Could you check a few things on this model? Use its own coordinates, in mm. A direction names the side the tool comes from. Give positions to 0.01 mm unless a question says otherwise; leave off trailing zeros. Write each loop counter-clockwise with the first axis right and the second up, starting at its lowest first coordinate (ties: lowest second). Pieces come first, ordered by that corner, then holes. Notation, with made-up numbers: M 24.25,-5 L 75.25,-5 A23 ccw 75.25,3 Z; hole C 88.5,-5 d3. An arc over 180 degrees is marked long. Answer as a JSON object with one key per item and string values. Group by question number.
```python
from build123d import *

# Parameters (mm, degrees)
F0_R        = 10.16
F1_DEPTH    = 3.81
F2_R        = 12.7
F3_DEPTH    = 2.54
F4_R        = 11.43
F5_DEPTH    = 38.1
F6_S5_R     = 12.7
F6_T6_DEPTH = 25
F7_W        = 12.7
F7_H        = 12.7
F8_DEPTH    = 16.51
F9_W        = 12.7
F9_H        = 12.7
F10_DEPTH   = 16.51


# Not quite as in the source:
# - a fillet or chamfer that OpenCascade refuses, or shapes differently, is made with other operations: its cross-section is extruded or revolved along the edge and cut away or added


with BuildPart() as f1:
    # F0 (on Top) → F1 (new body)
    with BuildSketch(Plane.XY):
        Circle(F0_R)
    extrude(amount=-F1_DEPTH)

    # F2 (on Top) → F3 (join)
    with BuildSketch(Plane.XY):
        Circle(F2_R)
    extrude(amount=F3_DEPTH)

    # F4 (on Top) → F5 (join)
    with BuildSketch(Plane.XY):
        Circle(F4_R)
    extrude(amount=F5_DEPTH)

    # F6: chamfer of 5.08 on 3 edges, made by hand


with BuildPart() as f6_tool2:
    # F6_s3 → F6_t4 (revolve)
    with BuildSketch(Plane.XZ):
        Polygon((16.51, 2.54), (11.43, 7.62), (11.43, 2.54), align=None)
    revolve(axis=Axis((0, 0, 2.54), (0, 0, -1)))

    # F6_s5 → F6_t6 (intersect, symmetric)
    with BuildSketch(Plane.XY.offset(5.1)):
        Circle(F6_S5_R)
    extrude(amount=F6_T6_DEPTH, both=True, mode=Mode.INTERSECT)


with BuildPart() as f1_1:
    add(f1.part)

    # F6_t1: union F6_tool2
    add(f6_tool2.part)

    # F6_s7 → F6_t8 (revolve, cut)
    with BuildSketch(Plane.XZ):
        Polygon((11.43, 33.02), (6.35, 38.1), (11.43, 38.1), align=None)
    revolve(axis=Axis((0, 0, 38.1), (0, 0, 1)), mode=Mode.SUBTRACT)

    # F7 (on Right) → F8 (join)
    with BuildSketch(Plane.YZ):
        with Locations((0, 19.9612583965)):
            Rectangle(F7_W, F7_H)
    extrude(amount=F8_DEPTH)

    # F9 (on Right) → F10 (join)
    with BuildSketch(Plane.YZ):
        with Locations((0, 19.9612583965)):
            Rectangle(F9_W, F9_H)
    extrude(amount=-F10_DEPTH)


solid = f1_1.part
```
1) If we section it at C-C, the plane z = 5.5: List the corners of the cut face in (x, y) for me, plus the area to 3 significant figures.
2) If we section it at B-B, the plane y = 0: List the corners of the cut face in (x, z) for me, plus the area to 3 significant figures.
3) I'm going to push flat-ended pins straight in: pin 1 (2 mm diameter, centred on y = -5.5, z = 7.5, fed in from +X); pin 2 (2 mm diameter, centred on x = -2.5, z = 16.5, fed in from -Y); pin 3 (2 mm diameter, centred on x = -13.5, y = -2, fed in from -Z). Where does each tip first touch, or does it pass through?
4) For faces 1 (the flat face through (-6, 9, 0)), 2 (the flat face through (13, -6.35, 20)), 3 (the flat face through (13, 6.35, 20)), 4 (the flat face through (-13, 6.35, 20)), which set-ups out of +Z, -Z, +X, -X, +Y, -Y let a thin tool reach every point of the face, with its end or its side?
5) If we section it at A-A, the plane x = 0: List the corners of the cut face in (y, z) for me, plus the area to 3 significant figures.
6) We'd pull the mould along Z, two halves only. Please class faces 5 (the flat face through (14, 0, 13.611)), 6 (the flat face through (-14, 0, 13.611)), 7 (the flat face through (-13, -6.35, 20)), 8 (the flat face through (14, 0, 26.311)): released by +Z, released by -Z, zero draft, split by the parting line, or undercut.
7) Please list where these lines run through material, in increasing order: line 1 along Y through (x, z) = (-14, 22.5); line 2 along Z through (x, y) = (10, 5.75); line 3 along X through (y, z) = (-2, 31). Write a range as from..to.
Taken from the geometry:
{
 "1": {"outline": "C 0,0 d25.4", "area": "507 mm²"},
 "2": {"outline": "M -16.51,13.61 L -11.43,13.61 L -11.43,7.62 L -12.7,6.35 L -12.7,0 L -10.16,0 L -10.16,-3.81 L 10.16,-3.81 L 10.16,0 L 12.7,0 L 12.7,6.35 L 11.43,7.62 L 11.43,13.61 L 16.51,13.61 L 16.51,26.31 L 11.43,26.31 L 11.43,33.02 L 6.35,38.1 L -6.35,38.1 L -11.43,33.02 L -11.43,26.31 L -16.51,26.31 Z", "area": "1,070 mm²"},
 "3": {"pin 1": "x = 11.38", "pin 2": "y = -11.33", "pin 3": "z = 0"},
 "4": {"face 1": "-Z", "face 2": "+Z, +X, -Y", "face 3": "+Z, +X, +Y", "face 4": "+Z, -X, +Y"},
 "5": {"outline": "M -12.7,0 L -10.16,0 L -10.16,-3.81 L 10.16,-3.81 L 10.16,0 L 12.7,0 L 12.7,6.35 L 11.43,7.62 L 11.43,33.02 L 6.35,38.1 L -6.35,38.1 L -11.43,33.02 L -11.43,7.62 L -12.7,6.35 Z", "area": "940 mm²"},
 "6": {"face 5": "undercut", "face 6": "undercut", "face 7": "zero draft", "face 8": "released by +Z"},
 "7": {"line 1": "-6.35..6.35", "line 2": "0..7.51, 13.61..26.31", "line 3": "-11.25..11.25"}
}
